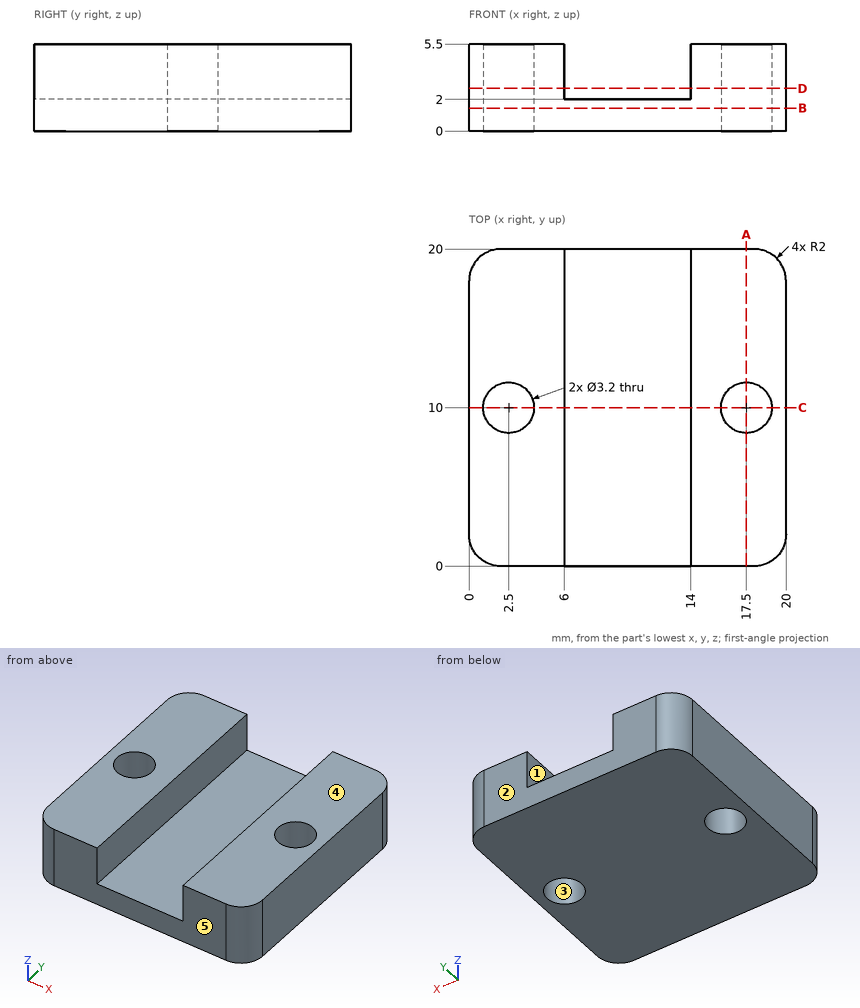
Part print with two shaded views. Sizes in mm from the minimum x, y, z corner. A direction names the side the tool comes from. Round coordinates to 2 decimals unless told otherwise and drop trailing zeros. Order: outer loops, then holes, each group sorted by start corner. A loop starts at its lowest first (then second) coordinate and runs counter-clockwise, first axis right, second up.
(1) 3-axis set-ups, long thin cutter, end or side, ignore diameter. For the marked faces 1 and 2: which of +Z, -Z, +X, -X, +Y, -Y reach the whole face in a straight line?
(2) Band-saw the part on B-B (z = 1.45). List the corners of the cut face in (x, y).
(3) Band-saw the part on D-D (z = 2.7). List the corners of the cut face in (x, y), then the cut area to 3 significant figures.
(4) Pin check, flat tip, straight feed: pin 1 (2 mm diameter, centred on x = 10.5, y = 10, fed in from +Z). Stop position of the tip, or through.
(5) Pull direction Y, two halves, no side cores. Call the marked faces 3, 4 and 5: released by +Y, released by -Y, zero draft, split by the parting line, or undercut.
(6) Band-saw the part on C-C (y = 10). List the corners of the cut face in (x, z), then the cut area to 3 significant figures.
(7) Drill centre lines: line 1 (X direction, y = 6.25, z = 3.75); line 2 (Y direction, x = 2.5, z = 2); line 3 (Y direction, x = 17, z = 3.35). Where is each one in solid material? Low to high.
(8) Band-saw the part on A-A (x = 17.5). List the corners of the cut face in (y, z), then the cut area to 3 significant figures.
Verdict:
1. face 1: +Z, +Y, -Y
1. face 2: +Z, -Z, +X, -X, +Y
2. outline: (0, 2) arc R2 ccw to (2, 0) - (18, 0) arc R2 ccw to (20, 2) - (20, 18) arc R2 ccw to (18, 20) - (2, 20) arc R2 ccw to (0, 18) - close; hole circle Ø3.2 at (2.5, 10); hole circle Ø3.2 at (17.5, 10)
3. outline: (0, 2) arc R2 ccw to (2, 0) - (6, 0) - (6, 20) - (2, 20) arc R2 ccw to (0, 18) - close; (14, 0) - (18, 0) arc R2 ccw to (20, 2) - (20, 18) arc R2 ccw to (18, 20) - (14, 20) - close; hole circle Ø3.2 at (2.5, 10); hole circle Ø3.2 at (17.5, 10)
3. area: 220 mm2
4. pin 1: stops at z = 2
5. face 3: undercut
5. face 4: zero draft
5. face 5: released by -Y
6. outline: (0, 0) - (0.9, 0) - (0.9, 5.5) - (0, 5.5) - close; (4.1, 0) - (15.9, 0) - (15.9, 5.5) - (14, 5.5) - (14, 2) - (6, 2) - (6, 5.5) - (4.1, 5.5) - close; (19.1, 0) - (20, 0) - (20, 5.5) - (19.1, 5.5) - close
6. area: 46.8 mm2
7. line 1: x = 0 to 6, 14 to 20
7. line 2: y = 0 to 8.4, 11.6 to 20
7. line 3: y = 0 to 8.48, 11.52 to 20
8. outline: (0, 0) - (8.4, 0) - (8.4, 5.5) - (0, 5.5) - close; (11.6, 0) - (20, 0) - (20, 5.5) - (11.6, 5.5) - close
8. area: 92.4 mm2
